```python
from build123d import *

# Parameters (mm, degrees)
BOSS_EXTRUDE1_DEPTH = 1.3
SKETCH3_W           = 1.22
SKETCH3_H           = 0.25
CUT_EXTRUDE1_DEPTH  = 0.17
CUT_EXTRUDE2_DEPTH  = 0.17
CUT_EXTRUDE3_DEPTH  = 0.1
SKETCH6_W           = 2.565
SKETCH6_H           = 1.079999998
SKETCH6_W_2         = 2.605000011
SKETCH6_H_2         = 1.079999997
CUT_EXTRUDE4_DEPTH  = 0.15
CUT_EXTRUDE5_DEPTH  = 0.95
SKETCH8_W           = 0.405
SKETCH8_H           = 7.3
BOSS_EXTRUDE2_DEPTH = 0.15
FILLET1_R           = 0.3
SKETCH9_W           = 0.44
SKETCH9_H           = 2.72
CUT_EXTRUDE6_DEPTH  = 0.15
LPATTERN1_COUNT     = 8
LPATTERN1_PITCH     = 1.1


with BuildPart() as part:
    # Sketch2 → Boss-Extrude1 (new body)
    with BuildSketch(Plane.XY):
        with BuildLine():
            Line((5.855, 5.140000001), (4.635, 5.140000001))
            Line((4.635, 5.140000001), (-5.02, 5.140000001))
            Line((-5.02, 5.140000001), (-5.02, 4.640000001))
            ThreePointArc((-5.02, 4.640000001), (-5.078578644, 4.498578644), (-5.22, 4.440000001))
            Line((-5.22, 4.440000001), (-5.855, 4.440000001))
            Line((-5.855, 4.440000001), (-5.855, -5.139999999))
            Line((-5.855, -5.139999999), (-5.205000011, -5.139999999))
            Line((-5.205000011, -5.139999999), (-2.6, -5.139999999))
            Line((-2.6, -5.139999999), (1.17, -5.139999999))
            Line((1.17, -5.139999999), (3.735, -5.139999999))
            Line((3.735, -5.139999999), (5.855, -5.139999999))
            Line((5.855, -5.139999999), (5.855, -4.659999975))
            Line((5.855, -4.659999975), (5.855, -3.259999975))
            Line((5.855, -3.259999975), (5.855, -1.150000033))
            Line((5.855, -1.150000033), (5.855, 0.439999967))
            Line((5.855, 0.439999967), (5.855, 4.890000001))
            Line((5.855, 4.890000001), (5.855, 5.140000001))
        make_face()
    extrude(amount=BOSS_EXTRUDE1_DEPTH)

    # Sketch3 → Cut-Extrude1 (cut)
    with BuildSketch(Plane(origin=(0, 0, 0), x_dir=(-1, 0, 0), z_dir=(0, 0, -1))):
        with Locations((-5.245, 5.015000001)):
            Rectangle(SKETCH3_W, SKETCH3_H)
    extrude(amount=-CUT_EXTRUDE1_DEPTH, mode=Mode.SUBTRACT)

    # Sketch4 → Cut-Extrude2 (cut)
    with BuildSketch(Plane(origin=(0, 0, 0), x_dir=(-1, 0, 0), z_dir=(0, 0, -1))):
        with BuildLine():
            Line((-5.855, -3.259999975), (-5.190000002, -3.259999975))
            ThreePointArc((-5.190000002, -3.259999975), (-5.013223307, -3.333223279), (-4.940000002, -3.509999975))
            Line((-4.940000002, -3.509999975), (-4.940000002, -4.409999975))
            ThreePointArc((-4.940000002, -4.409999975), (-5.013223307, -4.58677667), (-5.190000002, -4.659999975))
            Line((-5.190000002, -4.659999975), (-5.855, -4.659999975))
            Line((-5.855, -4.659999975), (-5.855, -3.259999975))
        make_face()
        Polygon((-4.455, -4.649999999), (-4.685, -4.649999999), (-4.845000002, -1.660000037), (-4.845000002, -1.150000033), (-5.855, -1.150000033), (-5.855, 0.439999967), (-4.865000002, 0.439999967), (-4.865000002, -0.110000037), (-4.455, -0.110000037), align=None)
    extrude(amount=-CUT_EXTRUDE2_DEPTH, mode=Mode.SUBTRACT)

    # Sketch5 → Cut-Extrude3 (cut)
    with BuildSketch(Plane(origin=(0, 0, 0), x_dir=(-1, 0, 0), z_dir=(0, 0, -1))):
        Polygon((5.205000011, -5.139999999), (2.6, -5.139999999), (-1.17, -5.139999999), (-3.735, -5.139999999), (-3.735, -4.060000001), (-3.735, -2.254355959), (-3.735, 1.690000007), (5.205000011, 1.690000007), (5.205000011, -2.080000002), (5.205000011, -4.060000002), align=None)
    extrude(amount=-CUT_EXTRUDE3_DEPTH, mode=Mode.SUBTRACT)

    # Sketch6 → Cut-Extrude4 (cut)
    with BuildSketch(Plane(origin=(0, 0, 0.1), x_dir=(-1, 0, 0), z_dir=(0, 0, -1))):
        with Locations((-2.4525, -4.6)):
            Rectangle(SKETCH6_W, SKETCH6_H)
        with Locations((3.902500006, -4.600000001)):
            Rectangle(SKETCH6_W_2, SKETCH6_H_2)
        with BuildLine():
            Line((5.205000011, 1.690000007), (5.205000011, -2.080000002))
            ThreePointArc((5.205000011, -2.080000002), (5.087842724, -2.362842714), (4.805000011, -2.480000002))
            Line((4.805000011, -2.480000002), (-3.375, -2.480000002))
            ThreePointArc((-3.375, -2.480000002), (-3.587435422, -2.41892653), (-3.735, -2.254355959))
            Line((-3.735, -2.254355959), (-3.735, 1.690000007))
            Line((-3.735, 1.690000007), (5.205000011, 1.690000007))
        make_face()
    extrude(amount=-CUT_EXTRUDE4_DEPTH, mode=Mode.SUBTRACT)


with BuildPart() as body_2:
    # Mirror1: mirrored copy
    add(part.part.mirror(Plane(origin=(-5.855, 4.440000001, 1.3), x_dir=(0, 0, 1), z_dir=(1, 0, 0))))

    # Sketch7 → Cut-Extrude5 (cut)
    with BuildSketch(Plane.XY.offset(1.3)):
        Polygon((-6.085, -2.859999999), (-16.345, -2.859999999), (-16.345, 5.140000001), (-16.345, 5.61631281), (-6.085, 5.61631281), align=None)
    extrude(amount=-CUT_EXTRUDE5_DEPTH, mode=Mode.SUBTRACT)

    # Sketch8 → Boss-Extrude2 (add)
    with BuildSketch(Plane.XY.offset(0.35)):
        with Locations((-6.2875, 0.790000001)):
            Rectangle(SKETCH8_W, SKETCH8_H)
    extrude(amount=BOSS_EXTRUDE2_DEPTH)

    # Fillet1
    fillet1_edges = [body_2.edges().sort_by_distance(p)[0] for p in [
        (-16.345, 1.140000001, 0.35),
    ]]
    fillet(fillet1_edges, radius=FILLET1_R)

    # Sketch9 → Cut-Extrude6 (cut)
    with BuildSketch(Plane.XY.offset(0.35)):
        with Locations((-7.115, 3.780000001)):
            Rectangle(SKETCH9_W, SKETCH9_H)
    cut_extrude6 = extrude(amount=-CUT_EXTRUDE6_DEPTH, mode=Mode.SUBTRACT)

    # LPattern1: Cut-Extrude6 ×8
    with Locations(*[(-i * LPATTERN1_PITCH, 0, 0) for i in range(1, LPATTERN1_COUNT)]):
        add(cut_extrude6, mode=Mode.SUBTRACT)


solid = body_2.part
```
Geometry: final body of the model. Coordinates: model frame, mm. A direction names the side the tool comes from. Round coordinates to 2 decimals unless told otherwise and drop trailing zeros. Order: outer loops, then holes, each group sorted by start corner. A loop starts at its lowest first (then second) coordinate and runs counter-clockwise, first axis right, second up. Notation, with made-up numbers: (40.25, -13.75) -> (56.25, -13.75) arc R22 cw to (56.25, -3.75) -> close; hole circle Ø8 at (37.25, 54). An arc over 180 degrees is marked (long way). Use CSV: the item, a comma, the result in double quotes. Start each with the question number.
1) Material intervals for line 1 along Y through (x, z) = (-17, 0.1); line 2 along X through (y, z) = (2.25, 1.1) (3 decimals); line 3 along Y through (x, z) = (-15.75, 0.8), sorted ascending. Write a range as from..to.
2) Draft query along Y for faces 1 (the face through (-11, -4, 0.1)), 2 (the face through (-17, -1, 0.17)), 3 (the face through (-13, 5.14, 0.2)). Return one class per face: +Y half, -Y half, draft (parallel to the pull), parting line (faces both ways), or undercut.
3) Section A-A (x = -8.75). Return the cut outline in (y, z), and give its area (3 significant figures).
4) Section B-B (y = -0.25). Return the cut outline in (x, z) (3 decimals).
5) Set-up query: faces 4 (the face through (-14.2, -4.6, 0.25)), 5 (the face through (-11, 2, 0.35)), 6 (the face through (-5.855, 0, 1)), 7 (the face through (-17, -4, 0.17)). Return all of +Z, -Z, +X, -X, +Y, -Y with unobstructed straight access to the full face (end or side cutting, diameter ignored); none if empty.
6) First-contact query: pin 1 Ø0.5 at (x, y) = (-9.5, 4) entering from +Z; pin 2 Ø6 at (x, y) = (-10.5, 3) entering from +Z. Flat tips, straight axial feed; report the tip coordinate or a pass-through.
7) Section D-D (x = -14.75). Return the cut outline in (y, z), and give its area (3 significant figures).
8) Section C-C (z = 1.1). Return the cut outline in (x, y) (3 decimals).
Returned:
1,line 1,"y = -5.14..-4.66, -3.26..-1.15, 0.44..4.89"
1,line 2,"x = -17.565..-16.345, -6.085..-5.855"
1,line 3,"y = -5.14..-2.86"
2,face 1,"draft"
2,face 2,"undercut"
2,face 3,"+Y half"
3,outline,"(-5.14, 0.25) -> (-4.06, 0.25) -> (-4.06, 0.1) -> (-2.48, 0.1) -> (-2.48, 0.25) -> (1.69, 0.25) -> (1.69, 0) -> (5.14, 0) -> (5.14, 0.35) -> (-2.86, 0.35) -> (-2.86, 1.3) -> (-5.14, 1.3) -> close"
3,area,"4.29 mm²"
4,outline,"(-17.565, 0.17) -> (-16.165, 0.17) -> (-16.165, 0) -> (-15.445, 0) -> (-15.445, 0.25) -> (-6.505, 0.25) -> (-6.505, 0) -> (-5.855, 0) -> (-5.855, 1.3) -> (-6.085, 1.3) -> (-6.085, 0.5) -> (-6.49, 0.5) -> (-6.49, 0.35) -> (-16.045, 0.35) arc R0.3 cw to (-16.345, 0.65) -> (-16.345, 1.3) -> (-17.565, 1.3) -> close"
5,face 4,"-Z, -Y"
5,face 5,"+Z, +Y"
5,face 6,"+Z, -Z, +X, +Y, -Y"
5,face 7,"-Z, -X"
6,pin 1,"stops at z = 0.35"
6,pin 2,"stops at z = 0.35"
7,outline,"(-5.14, 0.25) -> (-4.06, 0.25) -> (-4.06, 0.1) -> (-2.48, 0.1) -> (-2.48, 0.25) -> (1.69, 0.25) -> (1.69, 0) -> (5.14, 0) -> (5.14, 0.2) -> (2.42, 0.2) -> (2.42, 0.35) -> (-2.86, 0.35) -> (-2.86, 1.3) -> (-5.14, 1.3) -> close"
7,area,"3.89 mm²"
8,outline,"(-17.565, -5.14) -> (-5.855, -5.14) -> (-5.855, 4.44) -> (-6.085, 4.44) -> (-6.085, -2.86) -> (-16.345, -2.86) -> (-16.345, 5.14) -> (-17.565, 5.14) -> close"
